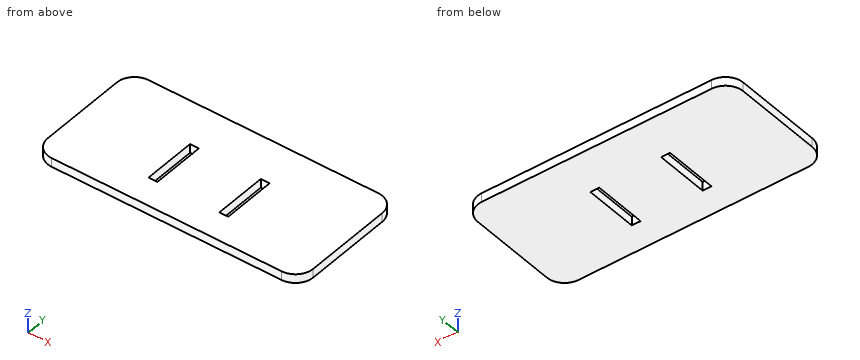
```python
from build123d import *

# Parameters (mm, degrees)
BOSS_EXTRUDE1_DEPTH = 10
SKETCH2_W           = 10
SKETCH2_H           = 60
CUT_EXTRUDE1_DEPTH  = 10


with BuildPart() as part:
    # Sketch1 → Boss-Extrude1 (new body)
    with BuildSketch(Plane.XY):
        with BuildLine():
            Line((80, 40), (-180, 40))
            ThreePointArc((-180, 40), (-194.142135624, 34.142135624), (-200, 20))
            Line((-200, 20), (-200, -80))
            ThreePointArc((-200, -80), (-194.142135624, -94.142135624), (-180, -100))
            Line((-180, -100), (80, -100))
            ThreePointArc((80, -100), (94.142135624, -94.142135624), (100, -80))
            Line((100, -80), (100, 20))
            ThreePointArc((100, 20), (94.142135624, 34.142135624), (80, 40))
        make_face()
    extrude(amount=BOSS_EXTRUDE1_DEPTH)

    # Sketch2 → Cut-Extrude1 (cut)
    with BuildSketch(Plane.XY.offset(10)):
        with Locations((-90, -38.5)):
            Rectangle(SKETCH2_W, SKETCH2_H)
        with Locations((-10, -38.5)):
            Rectangle(SKETCH2_W, SKETCH2_H)
    extrude(amount=-CUT_EXTRUDE1_DEPTH, mode=Mode.SUBTRACT)


solid = part.part
```
Can you work these out from the model? Positions are in its coordinate system, mm. Round coordinates to 2 decimals unless told otherwise and drop trailing zeros. Order: outer loops, then holes, each group sorted by start corner. A loop starts at its lowest first (then second) coordinate and runs counter-clockwise, first axis right, second up.
(1) If I drill on L1, parallel to X at y = -39, z = 5.5; L2, parallel to Y at x = -8, z = 4.75; L3, parallel to X at y = 21, z = 7.75, over which ranges is the centre line in solid material (lowest first)?
Results are:
L1: x = -200 to -95, -85 to -15, -5 to 100
L2: y = -100 to -68.5, -8.5 to 40
L3: x = -199.97 to 99.97
(2) I'm going to push a flat-ended pin straight in: pin 1 (4 mm diameter, centred on x = -120.5, y = -53, fed in from -Z). Where does the tip first touch, or does it pass through?
Results are:
pin 1: stops at z = 0
(3) If we section it at A-A (z = 5.25): Please give me the cut outline in (x, y), plus the area to 3 significant figures.
Results are:
outline: (-200, -80) arc R20 ccw to (-180, -100) - (80, -100) arc R20 ccw to (100, -80) - (100, 20) arc R20 ccw to (80, 40) - (-180, 40) arc R20 ccw to (-200, 20) - close; hole (-95, -68.5) - (-85, -68.5) - (-85, -8.5) - (-95, -8.5) - close; hole (-15, -68.5) - (-5, -68.5) - (-5, -8.5) - (-15, -8.5) - close
area: 40,500 mm2
